Here's how the part is built. I have some questions about the finished solid (model axes, mm). A direction names the side the tool comes from. Give positions to 0.01 mm unless a question says otherwise; leave off trailing zeros. Write each loop counter-clockwise with the first axis right and the second up, starting at its lowest first coordinate (ties: lowest second). Pieces come first, ordered by that corner, then holes. Notation, with made-up numbers: (-6.5, 79.25) -> (25.5, 79.25) arc R34 ccw to (25.5, 114.25) -> close; hole circle Ø4 at (85, -25). An arc over 180 degrees is marked (long way). Put each result on its own line as item: value. Start each with the question number.
from build123d import *

# Parameters (mm, degrees)
SKETCH1_R           = 20
BOSS_EXTRUDE1_DEPTH = 5
SKETCH2_R           = 1.6
CUT_EXTRUDE1_DEPTH  = 29.722813233
SKETCH3_R           = 9
BOSS_EXTRUDE2_DEPTH = 13
CUT_EXTRUDE2_DEPTH  = 34.526109228
CHAMFER3_SIZE       = 2
CHAMFER4_SIZE       = 1
CHAMFER5_SIZE       = 1
CHAMFER6_SIZE       = 0.5
CUT_EXTRUDE7_DEPTH  = 1.5


with BuildPart() as part:
    # Sketch1 → Boss-Extrude1 (new body)
    with BuildSketch(Plane(origin=(0, 0, 0), x_dir=(1, 0, 0), z_dir=(0, 1, 0))):
        with Locations(Location((0, 0, 0), (0, 0, 270))):
            Circle(SKETCH1_R)
    extrude(amount=BOSS_EXTRUDE1_DEPTH)

    # Sketch2 → Cut-Extrude1 (cut, through all)
    with BuildSketch(Plane(origin=(0, 5, 0), x_dir=(1, 0, 0), z_dir=(0, 1, 0))):
        with Locations(Location((0, 15, 0), (0, 0, 270))):
            Circle(SKETCH2_R)
        with Locations(Location((12.990381057, 7.5, 0), (0, 0, 270))):
            Circle(SKETCH2_R)
        with Locations(Location((12.990381057, -7.5, 0), (0, 0, 270))):
            Circle(SKETCH2_R)
        with Locations(Location((0, -15, 0), (0, 0, 270))):
            Circle(SKETCH2_R)
        with Locations(Location((-12.990381057, -7.5, 0), (0, 0, 270))):
            Circle(SKETCH2_R)
        with Locations(Location((-12.990381057, 7.5, 0), (0, 0, 270))):
            Circle(SKETCH2_R)
    extrude(amount=-CUT_EXTRUDE1_DEPTH, mode=Mode.SUBTRACT)

    # Sketch3 → Boss-Extrude2 (add)
    with BuildSketch(Plane(origin=(0, 5, 0), x_dir=(1, 0, 0), z_dir=(0, 1, 0))):
        with Locations(Location((0, 0, 0), (0, 0, 90))):
            Circle(SKETCH3_R)
    extrude(amount=BOSS_EXTRUDE2_DEPTH)

    # Sketch4 → Cut-Extrude2 (cut, through all)
    with BuildSketch(Plane(origin=(0, 18, 0), x_dir=(1, 0, 0), z_dir=(0, 1, 0))):
        with BuildLine():
            Line((1.754992877, 2.525), (-1.754992877, 2.525))
            ThreePointArc((-1.754992877, 2.525), (-1.424609052, -2.725089732), (3.075, 0))
            ThreePointArc((3.075, 0), (2.725089732, 1.424609052), (1.754992877, 2.525))
        make_face()
    extrude(amount=-CUT_EXTRUDE2_DEPTH, mode=Mode.SUBTRACT)

    # Chamfer3
    chamfer3_edges = [part.edges().sort_by_distance(p)[0] for p in [
        (0, 5, 9),
    ]]
    chamfer(chamfer3_edges, length=CHAMFER3_SIZE)

    # Chamfer4
    chamfer4_edges = [part.edges().sort_by_distance(p)[0] for p in [
        (0, 5, -20),
    ]]
    chamfer(chamfer4_edges, length=CHAMFER4_SIZE)

    # Chamfer5
    chamfer5_edges = [part.edges().sort_by_distance(p)[0] for p in [
        (0, 18, 9),
    ]]
    chamfer(chamfer5_edges, length=CHAMFER5_SIZE)

    # Chamfer6
    chamfer6_edges = [part.edges().sort_by_distance(p)[0] for p in [
        (0, 18, -2.525),
        (0, 18, 3.075),
    ]]
    chamfer(chamfer6_edges, length=CHAMFER6_SIZE)

    # Sketch10 → Cut-Extrude7 (cut)
    with BuildSketch(Plane(origin=(0, 5, 0), x_dir=(1, 0, 0), z_dir=(0, 1, 0))):
        Polygon((1.645448267, 17.85), (-1.645448267, 17.85), (-3.290896534, 15), (-1.645448267, 12.15), (1.645448267, 12.15), (3.290896534, 15), align=None)
        Polygon((14.635829324, 10.35), (11.34493279, 10.35), (9.699484522, 7.5), (11.34493279, 4.65), (14.635829324, 4.65), (16.281277591, 7.5), align=None)
        Polygon((-11.34493279, 10.35), (-14.635829324, 10.35), (-16.281277591, 7.5), (-14.635829324, 4.65), (-11.34493279, 4.65), (-9.699484522, 7.5), align=None)
    cut_extrude7 = extrude(amount=-CUT_EXTRUDE7_DEPTH, mode=Mode.SUBTRACT)

    # Mirror2: Cut-Extrude7 across plane
    add(cut_extrude7.mirror(Plane.XY), mode=Mode.SUBTRACT)


solid = part.part
1) I want a section at A-A, the plane y = 9.75. Write out the boundary of the cut face in (x, z) (3 decimals).
2) I want a section at B-B, the plane x = 0. State how many separate pieces and enclosed holes the cut face has, and give its area (3 significant figures).
3) I need wall thicknesses on probe 1 along X at (y, z) = (1.5, 6.5); probe 2 along X at (y, z) = (1.15, -7.5); probe 3 along Z at (x, y) = (-14, 4.25). Which ranges of each line are inside material? Lowest first, please.
4) Which directions (+Z, -Z, +X, -X, +Y, -Y) give clear straight access to the entire face, cutting with the end or side of a thin tool? Please do faces 4 (the flat face through (0, 4, 17.85)), 5 (the cylindrical face through (0.07, 1.77, 13.4)).
5) Thinking about a two-plate mould opening in X: for faces 1 (the flat face through (-0.1, 18, -3.4)), 2 (the cylindrical face through (-2.703, 11.93, -8.584)), 3 (the flat face through (15.47, 4.26, 8.905)), which applies, released by +X, released by -X, zero draft, split by the parting line, or undercut?
6) I'm going to push flat-ended pins straight in: pin 1 Ø0.8 at (x, y) = (-13, 4) entering from -Z; pin 2 Ø1.7 at (x, z) = (0.5, 16) entering from +Y; pin 3 Ø5 at (y, z) = (16, 2) entering from -X; pin 4 Ø12 at (x, z) = (0.5, -9) entering from +Y. Where does each tip first touch, or does it pass through?
Established:
1. outline: circle Ø18 at (0, 0); hole (-1.755, -2.525) -> (1.755, -2.525) arc R3.075 ccw (long way) to start
2. separate pieces: 4
2. enclosed holes: 0
2. area: 295 mm2
3. probe 1: x = -18.91 to -14.24, -11.74 to 11.74, 14.24 to 18.91
3. probe 2: x = -18.54 to -14.59, -11.39 to 11.39, 14.59 to 18.54
3. probe 3: z = -13.93 to -10.35, -4.65 to 4.65, 10.35 to 13.93
4. face 4: +Y
4. face 5: +Y, -Y
5. face 1: zero draft
5. face 2: split by the parting line
5. face 3: undercut
6. pin 1: stops at z = -15.53
6. pin 2: stops at y = 3.5
6. pin 3: stops at x = -9
6. pin 4: stops at y = 18
